Build history of the part. All positions in model axes, mm. Give positions to 0.01 mm unless a question says otherwise; leave off trailing zeros. Write each loop counter-clockwise with the first axis right and the second up, starting at its lowest first coordinate (ties: lowest second). Pieces come first, ordered by that corner, then holes.
from build123d import *

# Parameters (mm, degrees)
F0_W     = 172.279298
F0_H     = 81.796013
F1_DEPTH = 25.4
F3_D     = 19.05
F4_R     = 12.7


with BuildPart() as f1:
    # F0 (on Top) → F1 (new body)
    with BuildSketch(Plane.XY):
        with Locations((0, 40.898007)):
            Rectangle(F0_W, F0_H)
    extrude(amount=F1_DEPTH)

    # F3 (through all)
    with Locations(Plane.XY.offset(25.4)):
        with Locations((51.449351, 37.283532), (-59.726231, 49.170807)):
            Hole(F3_D / 2)

    # F4
    f4_edges = [f1.edges().sort_by_distance(p)[0] for p in [
        (0, 81.796013, 25.4),
        (-86.139649, 40.898006, 25.4),
        (0, 0, 25.4),
        (86.139649, 40.898006, 25.4),
    ]]
    fillet(f4_edges, radius=F4_R)


solid = f1.part
(1) Saw through at C-C, the plane z = 18. List the corners of the cut face in (x, y) (3 decimals).
(2) Probe line 1 (X direction, y = 48.5, z = 10.75); line 2 (X direction, y = 33.5, z = 22.25); line 3 (Y direction, x = -54.5, z = 14.25). List the from-to ranges inside material, lowest first.
(3) Saw through at B-B, the plane y = 43.5. List the corners of the cut face in (x, z).
(4) Saw through at A-A, the plane x = 54.5. List the corners of the cut face in (y, z), plus the area to 3 significant figures.
(5) Drop flat-ended pins along their axis: pin 1 (4 mm diameter, centred on y = 67, z = 20.5, fed in from +X); pin 2 (15 mm diameter, centred on x = 51.45, y = 37.28, fed in from -Z). Give the stop position or say it passes through.
(6) Saw through at D-D, the plane y = 54. List the corners of the cut face in (x, z).
(7) Mould opens along Y. For faces 1 (the face through (-52.17, 43.37, 12.52)), 2 (the face through (86.14, 40, 6)), 3 (the face through (52.689, 46.727, 12.522)), 4 (the face through (1.21, 3.62, 21.58)) say: +Y half, -Y half, draft (parallel to the pull), parting line (faces both ways), or undercut.
Computed values:
1. outline: (-84.981, 1.159) - (84.981, 1.159) - (84.981, 80.637) - (-84.981, 80.637) - close; hole circle Ø19.05 at (-59.726, 49.171); hole circle Ø19.05 at (51.449, 37.284)
2. line 1: x = -86.14 to -69.23, -50.22 to 86.14
2. line 2: x = -81.81 to 42.71, 60.19 to 81.81
2. line 3: y = 0.09 to 41.21, 57.13 to 81.7
3. outline: (-86.14, 0) - (-67.38, 0) - (-67.38, 25.4) - (-73.44, 25.4) arc R12.7 ccw to (-86.14, 12.7) - close; (-52.07, 0) - (44.23, 0) - (44.23, 25.4) - (-52.07, 25.4) - close; (58.67, 0) - (86.14, 0) - (86.14, 12.7) arc R12.7 ccw to (73.44, 25.4) - (58.67, 25.4) - close
4. outline: (0, 0) - (28.26, 0) - (28.26, 25.4) - (12.7, 25.4) arc R12.7 ccw to (0, 12.7) - close; (46.31, 0) - (81.8, 0) - (81.8, 12.7) arc R12.7 ccw to (69.1, 25.4) - (46.31, 25.4) - close
4. area: 1,550 mm2
5. pin 1: stops at x = 84.74
5. pin 2: passes through
6. outline: (-86.14, 0) - (-67.94, 0) - (-67.94, 25.4) - (-73.44, 25.4) arc R12.7 ccw to (-86.14, 12.7) - close; (-51.52, 0) - (86.14, 0) - (86.14, 12.7) arc R12.7 ccw to (73.44, 25.4) - (-51.52, 25.4) - close
7. face 1: undercut
7. face 2: draft
7. face 3: undercut
7. face 4: -Y half
